Verification items for the finished model (mm, model axes). Face numbers are marked on the shaded views. A direction names the side the tool comes from. Coordinates: 2 decimals unless noted, no trailing zeros. Order: outer loops, then holes, each group sorted by start corner. A loop starts at its lowest first (then second) coordinate and runs counter-clockwise, first axis right, second up. Notation, with made-up numbers: M 88.5,20.5 L 96.5,20.5 A20 cw 96.5,40.5 Z; hole C 12,-7 d1. An arc over 180 degrees is marked long. Write item = value, one per line.
Autodesk Fusion 360 part; units mm, degrees
sketch "Boceto1" plane through (0, 0, 0) normal (0, 0, 1) x (1, 0, 0)
  line L0 (0, 0) -> (80, 0) construction
  line L1 (80, 0) -> (80, 60) construction
  line L2 (80, 60) -> (0, 60) construction
  line L3 (0, 60) -> (0, 0) construction
  circle A0 centre (5, 55) radius 1.625
  circle A1 centre (75, 55) radius 1.625
  line L4 (110, -5) -> (-30, -5)
  line L5 (-30, -5) -> (-30, 65)
  line L6 (-30, 65) -> (110, 65)
  line L7 (110, 65) -> (110, -5)
  line L8 (15, 46) -> (65, 46)
  line L9 (65, 46) -> (65, 48)
  line L10 (65, 48) -> (15, 48)
  line L11 (15, 48) -> (15, 46)
  line L12 (-30, 30) -> (115, 30)
  line L13 (110, 30) -> (107, 30)
  line L14 (107, 30) -> (107, 44)
  line L15 (107, 44) -> (110, 44)
  line L16 (110, 44) -> (110, 30)
  line L17 (110, 16) -> (110, 30)
  line L18 (110, 30) -> (107, 30)
  line L19 (107, 16) -> (110, 16)
  line L20 (107, 30) -> (107, 16)
  line L21 (40, 65) -> (40, -5)
  circle A2 centre (5, 5) radius 1.625
  circle A3 centre (75, 5) radius 1.625
  line L22 (-30, 44) -> (-30, 30)
  line L23 (-30, 30) -> (-27, 30)
  line L24 (-27, 30) -> (-27, 44)
  line L25 (-27, 44) -> (-30, 44)
  line L26 (-30, 16) -> (-30, 30)
  line L27 (-30, 30) -> (-27, 30)
  line L28 (-27, 16) -> (-30, 16)
  line L29 (-27, 30) -> (-27, 16)
  line L30 (65, 12) -> (15, 12)
  line L31 (15, 12) -> (15, 14)
  line L32 (15, 14) -> (65, 14)
  line L33 (65, 14) -> (65, 12)
  dimension "d1" = 80
  dimension "d2" = 60
  dimension "d3" = 5
  dimension "d4" = 70
  dimension "d8" = 3.25
  dimension "d16" = 70
  dimension "d17" = 140
  dimension "d19" = 30
  dimension "d20" = 5
  dimension "d29" = 7
  dimension "d31" = 2
  dimension "d34" = 50
  dimension "d37" = 14
  dimension "d38" = 3
  dimension "d39" = 5
extrude "Extruir1" add sketch "Boceto1" along normal blind 5 contours L4 L7 L12 L19 L20 L21 L30 L32 L33 | L4 L5 L12 L21 L28 L29 L30 L31 L32 | L6 L7 L8 L9 L10 L12 L14 L15 L21 | L5 L6 L8 L10 L11 L12 L21 L24 L25
sketch "Boceto4" plane through (0, 0, 5) normal (0, 0, 1) x (-1, 0, 0)
  line L0 (-15, -14) -> (-65, -14)
  line L1 (-65, -14) -> (-65, -12)
  line L2 (-65, -12) -> (-15, -12)
  line L3 (-15, -12) -> (-15, -14)
  circle A0 centre (-5, -5) radius 1.625
  circle A1 centre (-75, -55) radius 1.625
  circle A2 centre (-75, -5) radius 1.625
  circle A3 centre (-5, -55) radius 1.625
  line L4 (-15, -46) -> (-15, -48)
  line L5 (-15, -48) -> (-65, -48)
  line L6 (-65, -48) -> (-65, -46)
  line L7 (-65, -46) -> (-15, -46)
  line L8 (27, -44) -> (27, -16)
  line L9 (27, -16) -> (30, -16)
  line L10 (30, -16) -> (30, 5)
  line L11 (30, 5) -> (-110, 5)
  line L12 (-110, 5) -> (-110, -16)
  line L13 (-110, -16) -> (-107, -16)
  line L14 (-107, -16) -> (-107, -44)
  line L15 (-107, -44) -> (-110, -44)
  line L16 (-110, -44) -> (-110, -65)
  line L17 (-110, -65) -> (30, -65)
  line L18 (30, -65) -> (30, -44)
  line L19 (30, -44) -> (27, -44)
  line L20 (-107, -44) -> (-103, -44)
  line L21 (-103, -44) -> (-103, -16)
  line L22 (-103, -16) -> (-107, -16)
  line L23 (-107, -16) -> (-107, -44)
  line L24 (-40, -65) -> (-40, 5)
  line L25 (27, -30) -> (-107, -30)
  line L26 (27, -16) -> (27, -44)
  line L27 (27, -44) -> (23, -44)
  line L28 (23, -44) -> (23, -16)
  line L29 (23, -16) -> (27, -16)
  circle A4 centre (-5, -55) radius 3
  circle A5 centre (-75, -55) radius 3
  circle A6 centre (-5, -5) radius 3
  circle A7 centre (-75, -5) radius 3
  dimension "d42" = 4
  dimension "d58" = 6
extrude "Extruir3" add sketch "Boceto4" along normal blind 20 contours L8 L25 L26 L28 L29 | L8 L25 L26 L27 L28 | L14 L21 L22 L23 L25 | L14 L20 L21 L23 L25
extrude "Extruir2" add sketch "Boceto4" along normal blind 10 contours L8 L25 L26 L28 L29 | L8 L25 L26 L27 L28 | L14 L21 L22 L23 L25 | L14 L20 L21 L23 L25
sketch "Boceto5" plane through (107, 0, 0) normal (1, 0, 0) x (0, 1, 0)
  line L0 (16, 0) -> (44, 0)
  line L1 (44, 0) -> (44, 5)
  line L2 (44, 5) -> (44, 25)
  line L3 (16, 25) -> (16, 5)
  line L4 (16, 5) -> (16, 0)
  line L5 (30, 25) -> (30, 0)
  line L6 (44, 25) -> (16, 25)
  line L7 (19.65, 21.5) -> (19.65, 9.5)
  arc A0 (19.65, 9.5) -> (22.85, 9.5) centre (21.25, 9.5) ccw
  line L8 (22.85, 9.5) -> (22.85, 21.5)
  arc A1 (22.85, 21.5) -> (19.65, 21.5) centre (21.25, 21.5) ccw
  line L9 (21.25, 21.5) -> (21.25, 9.5) construction
  arc A2 (37.15, 9.5) -> (40.35, 9.5) centre (38.75, 9.5) ccw
  line L10 (37.15, 9.5) -> (37.15, 21.5)
  arc A3 (40.35, 21.5) -> (37.15, 21.5) centre (38.75, 21.5) ccw
  line L11 (40.35, 21.5) -> (40.35, 9.5)
  dimension "d52" = 3.2
  dimension "d53" = 12
  dimension "d54" = 8.75
  dimension "d55" = 3.5
sketch "Boceto2" plane through (0, 0, 0) normal (0, 0, 1) x (1, 0, 0)
sketch "Boceto3" plane through (0, 0, 0) normal (0, 0, 1) x (1, 0, 0)
  point P0 (5, 55)
extrude "Extruir4" cut sketch "Boceto5" against normal blind 155 contours L7 A0 L8 A1 | A2 L10 A3 L11
extrude "Extruir5" add sketch "Boceto4" along normal blind 8 contours A4 | A5 | A6 | A7
sketch "Boceto6" plane through (0, 0, 5) normal (0, 0, 1) x (-1, 0, 0)
  line L0 (10, -30) -> (-10, -30)
  line L1 (-10, -30) -> (-10, -49)
  line L2 (-10, -49) -> (10, -49)
  line L3 (10, -49) -> (10, -30)
  line L4 (-15, -65) -> (-40, -65)
  line L5 (-40, -65) -> (-40, -52)
  line L6 (-40, -52) -> (-15, -52)
  line L7 (-15, -52) -> (-15, -65)
  line L8 (-40, -65) -> (-40, 5)
  line L9 (-90, -49) -> (-90, -30)
  line L10 (-90, -30) -> (-70, -30)
  line L11 (-70, -30) -> (-70, -49)
  line L12 (-70, -49) -> (-90, -49)
  line L13 (27, -30) -> (-107, -30)
  line L14 (-10, -30) -> (-10, -11)
  line L15 (-10, -11) -> (10, -11)
  line L16 (10, -11) -> (10, -30)
  line L17 (10, -30) -> (-10, -30)
  line L18 (-70, -30) -> (-70, -11)
  line L19 (-70, -11) -> (-90, -11)
  line L20 (-90, -11) -> (-90, -30)
  line L21 (-90, -30) -> (-70, -30)
  line L22 (-65, -65) -> (-40, -65)
  line L23 (-40, -65) -> (-40, -52)
  line L24 (-40, -52) -> (-65, -52)
  line L25 (-65, -52) -> (-65, -65)
  line L26 (-15, 5) -> (-40, 5)
  line L27 (-40, 5) -> (-40, -8)
  line L28 (-40, -8) -> (-15, -8)
  line L29 (-15, -8) -> (-15, 5)
  line L30 (-40, -8) -> (-65, -8)
  line L31 (-65, -8) -> (-65, 5)
  line L32 (-65, 5) -> (-40, 5)
  line L33 (-40, 5) -> (-40, -8)
  line L34 (-40, -30) -> (-16, -30)
  line L35 (-16, -30) -> (-16, -35)
  line L36 (-16, -35) -> (-40, -35)
  line L37 (-40, -35) -> (-40, -30)
  line L38 (-40, -30) -> (-64, -30)
  line L39 (-64, -30) -> (-64, -35)
  line L40 (-40, -35) -> (-40, -30)
  line L41 (-64, -35) -> (-40, -35)
  line L42 (-40, -30) -> (-16, -30)
  line L43 (-16, -30) -> (-16, -25)
  line L44 (-16, -25) -> (-40, -25)
  line L45 (-40, -25) -> (-40, -30)
  line L46 (-40, -30) -> (-64, -30)
  line L47 (-64, -30) -> (-64, -25)
  line L48 (-64, -25) -> (-40, -25)
  line L49 (-40, -25) -> (-40, -30)
  arc A0 (-103, 5) -> (-110, -2) centre (-103, -2) ccw
  line L50 (-103, 5) -> (-110, 5)
  line L51 (-110, 5) -> (-110, -2)
  line L52 (30, 5) -> (30, -2)
  line L53 (23, 5) -> (30, 5)
  arc A1 (30, -2) -> (23, 5) centre (23, -2) ccw
  line L54 (-110, -65) -> (-110, -58)
  line L55 (-103, -65) -> (-110, -65)
  arc A2 (-110, -58) -> (-103, -65) centre (-103, -58) ccw
  line L56 (30, -65) -> (30, -58)
  arc A3 (23, -65) -> (30, -58) centre (23, -58) ccw
  line L57 (23, -65) -> (30, -65)
  point P0 (-5, -55)
  point P1 (-75, -5)
  point P2 (-110, 5)
  dimension "d61" = 15
  dimension "d62" = 6
  dimension "d63" = 19
  dimension "d64" = 20
  dimension "d65" = 25
  dimension "d66" = 13
  dimension "d67" = 24
  dimension "d68" = 5
  dimension "d72" = 7
  dimension "d73" = 3
extrude "Extruir6" cut sketch "Boceto6" against normal blind 25 contours L0 L1 L2 L3 L13 L17 | L4 L5 L6 L7 L8 L23 | L5 L8 L22 L23 L24 L25 | L9 L10 L11 L12 L13 L21 | L10 L13 L18 L19 L20 L21 | L8 L27 L30 L31 L32 L33 | L8 L26 L27 L28 L29 L33 | L8 L13 L34 L35 L36 L37 L40 L42 | L8 L13 L34 L42 L43 L44 L45 L49 | L0 L13 L14 L15 L16 L17 | L8 L13 L38 L45 L46 L47 L48 L49 | L8 L13 L37 L38 L39 L40 L41 L46
extrude "Extruir7" cut sketch "Boceto6" against normal blind 15 contours A0 L50 L51 | L52 L53 A1 | L54 L55 A2 | L56 A3 L57
equation "d37 = ( 28 / 2 ) * 1 mm"
equation "d54 = ( 17.5 / 2 ) * 1 mm"
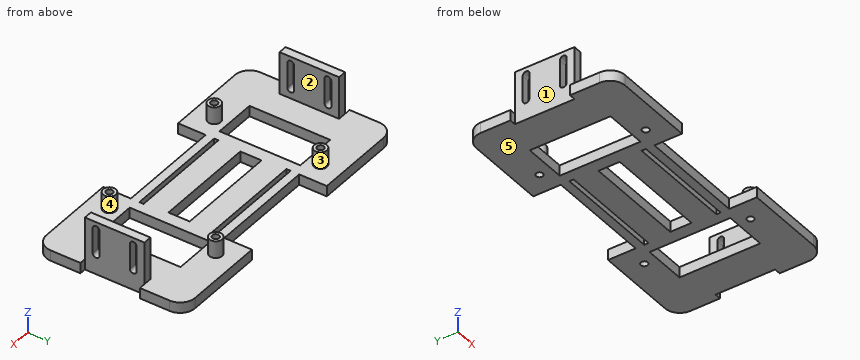
Item 1: Sectioned sample at C-C, the plane x = 21. Enter the section's corners in (y, z).
Report:
outline = M 8,0 L 12,0 L 12,5 L 8,5 Z; M 14,0 L 25,0 L 25,5 L 14,5 Z; M 35,0 L 46,0 L 46,5 L 35,5 Z; M 48,0 L 52,0 L 52,5 L 48,5 Z
Item 2: Gauge pin test, flat ends, axial feed: pin 1 (4.5 mm diameter, centred on x = 105.5, z = 17, fed in from -Y); pin 2 (1.5 mm diameter, centred on x = -28, z = 2, fed in from +Y); pin 3 (5.5 mm diameter, centred on y = 31.5, z = 3, fed in from +X). Record the tip position at first contact, or that the pin passes through.
Report:
pin_1 = 16
pin_2 = 63.56
pin_3 = 107
Item 3: Release check for a two-part mould opening along Y. For the marked faces 4 and 5 record: pulls with the +Y half, pulls with the -Y half, needs draft (parallel to the pull), parting line crosses it, or undercut.
Report:
face_4 = undercut
face_5 = needs draft
Item 4: Sectioned sample at A-A, the plane y = 27. Enter the section's corners in (x, z), then the cut area to 3 significant figures.
Report:
outline = M -27,0 L -10,0 L -10,5 L -23,5 L -23,25 L -27,25 Z; M 10,0 L 16,0 L 16,5 L 10,5 Z; M 64,0 L 70,0 L 70,5 L 64,5 Z; M 90,0 L 107,0 L 107,25 L 103,25 L 103,5 L 90,5 Z
area = 390 mm^2
Item 5: Scan lines: L1, parallel to Y at x = 75, z = 3.75 (3 decimals); L2, parallel to Y at x = 75, z = 6 (3 decimals); L3, parallel to X at y = 55, z = 5.25 (3 decimals). Record each from-to range of solid material in increasing order. Write a range as from..to.
Report:
L1 = -5..3.375, 6.625..11, 49..53.375, 56.625..65
L2 = 2..3.375, 6.625..8, 52..53.375, 56.625..58
L3 = 2..3.375, 6.625..8, 72..73.375, 76.625..78
Item 6: Sectioned sample at D-D, the plane y = 38.75. Enter the section's corners in (x, z).
Report:
outline = M -27,0 L -10,0 L -10,5 L -23,5 L -23,7.9 L -27,7.9 Z; M -27,23.1 L -23,23.1 L -23,25 L -27,25 Z; M 10,0 L 70,0 L 70,5 L 10,5 Z; M 90,0 L 107,0 L 107,7.9 L 103,7.9 L 103,5 L 90,5 Z; M 103,23.1 L 107,23.1 L 107,25 L 103,25 Z
Item 7: Tool access check on the marked faces 1, 2 and 3. Record the directions out of +Z, -Z, +X, -X, +Y, -Y that give a thin tool (end or side, any length) a straight path to the whole face; none if there is none.
Report:
face_1 = +Z, -Z, -X
face_2 = +Z, +Y, -Y
face_3 = +Z
